```python
from build123d import *

# Parameters (mm, degrees)
SKETCH1_R               = 11
SKETCH1_R_2             = 5
SKETCH1_R_3             = 1.5
BOSS_EXTRUDE1_DEPTH     = 2
SKETCH1_3_R             = 5
SKETCH1_3_R_2           = 2
BOSS_EXTRUDE2_DEPTH     = 12
CUT_EXTRUDE1_REACH      = 25.759
CUT_EXTRUDE1_END_RADIUS = 2
SKETCH2_R               = 1.5


with BuildPart() as part:
    # Sketch1 → Boss-Extrude1 (new body)
    with BuildSketch(Plane(origin=(0, 0, 0), x_dir=(1, 0, 0), z_dir=(0, 1, 0))):
        with Locations(Location((0, 0, 0), (0, 0, 270))):
            Circle(SKETCH1_R)
        with Locations(Location((0, 0, 0), (0, 0, 270))):
            Circle(SKETCH1_R_2, mode=Mode.SUBTRACT)
        with Locations(Location((0, 8, 0), (0, 0, 270))):
            Circle(SKETCH1_R_3, mode=Mode.SUBTRACT)
        with Locations(Location((8, 0, 0), (0, 0, 270))):
            Circle(SKETCH1_R_3, mode=Mode.SUBTRACT)
        with Locations(Location((0, -8, 0), (0, 0, 270))):
            Circle(SKETCH1_R_3, mode=Mode.SUBTRACT)
        with Locations(Location((-8, 0, 0), (0, 0, 270))):
            Circle(SKETCH1_R_3, mode=Mode.SUBTRACT)
    extrude(amount=BOSS_EXTRUDE1_DEPTH)

    # Sketch1_3 → Boss-Extrude2 (add)
    with BuildSketch(Plane(origin=(0, 0, 0), x_dir=(1, 0, 0), z_dir=(0, 1, 0))):
        with Locations(Location((0, 0, 0), (0, 0, 270))):
            Circle(SKETCH1_3_R)
        with Locations(Location((0, 0, 0), (0, 0, 270))):
            Circle(SKETCH1_3_R_2, mode=Mode.SUBTRACT)
    extrude(amount=BOSS_EXTRUDE2_DEPTH)

    # Cut-Extrude1: up to this cylinder (the profile starts outside it)
    cut_extrude1_end = Plane(origin=(0, 9, 0), z_dir=(0, -1, 0)) * Cylinder(CUT_EXTRUDE1_END_RADIUS, 56.518, mode=Mode.PRIVATE)
    # Sketch2 → Cut-Extrude1 (cut, up to the surface)
    with BuildSketch(Plane(origin=(-4.0625, 0, 2.914805954), x_dir=(0.582961190817979, 0, 0.8125000000000517), z_dir=(-0.8125000000000517, 0, 0.582961190817979)), mode=Mode.PRIVATE) as cut_extrude1_sk1:
        with Locations((0, 9)):
            Circle(SKETCH2_R)
    cut_extrude1_tool1 = extrude(cut_extrude1_sk1.sketch, amount=-CUT_EXTRUDE1_REACH, mode=Mode.PRIVATE) - cut_extrude1_end
    add(cut_extrude1_tool1.solids().sort_by_distance((-4.0625, 9, 2.914806))[0], mode=Mode.SUBTRACT)


solid = part.part
```
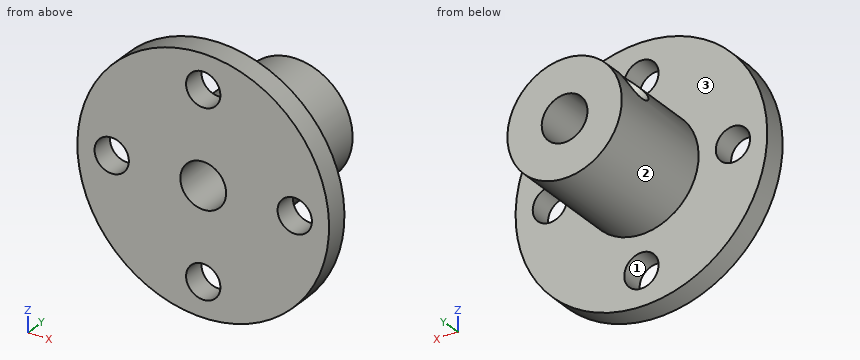
Can you work these out from the model? Positions are in its coordinate system, mm. Face numbers are marked on the shaded views. Coordinates: 2 decimals unless noted, no trailing zeros. Loops run counter-clockwise (first coordinate to the right, second up) from the corner with the lowest first, then second, coordinate; pieces in that order, holes last. Notation, with made-up numbers: M 59,-19 L 70,-19 A7 cw 70,-15 Z; hole C 46.25,50 d3. An arc over 180 degrees is marked long. Put each result on its own line as item: value. Start each with the question number.
(1) Imagine slicing it at A-A on x = 8. List the corners of the cut face in (y, z) for me, and give its area (3 significant figures).
(2) Imagine slicing it at B-B on z = 8. List the corners of the cut face in (x, y) for me, and give its area (3 significant figures).
(3) Imagine slicing it at C-C on y = 2.75. List the corners of the cut face in (x, z) for me, and give its area (3 significant figures).
(4) I need wall thicknesses on probe 1 along X at (y, z) = (1.05, 0); probe 2 along Y at (x, z) = (-5.5, 0.75); probe 3 along X at (y, z) = (0.4, 8). Which ranges of each line are inside material? Lowest first, please.
(5) Will these pins go through, and if not, where does the flat tip stop? pin 1 Ø3.5 at (x, z) = (0, 8) entering from +Y; pin 2 Ø4 at (x, y) = (-8, 2.5) entering from +Z; pin 3 Ø3 at (x, y) = (3, 10) entering from +Z.
(6) We'd pull the mould along X, two halves only. Please class the marked faces 1, 2 and 3: +X half, -X half, draft (parallel to the pull), parting line (faces both ways), or undercut.
(7) Imagine slicing it at D-D on z = -1. List the corners of the cut face in (x, y) for me.
Worked answers:
1. outline: M 0,-7.55 L 2,-7.55 L 2,-1.5 L 0,-1.5 Z; M 0,1.5 L 2,1.5 L 2,7.55 L 0,7.55 Z
1. area: 24.2 mm2
2. outline: M -7.55,0 L -1.5,0 L -1.5,2 L -7.55,2 Z; M 1.5,0 L 7.55,0 L 7.55,2 L 1.5,2 Z
2. area: 24.2 mm2
3. outline: C 0,0 d10; hole C 0,0 d4
3. area: 66.0 mm2
4. probe 1: x = -11 to -9.5, -6.5 to -2, 2 to 6.5, 9.5 to 11
4. probe 2: y = 0 to 2
4. probe 3: x = -7.55 to -1.5, 1.5 to 7.55
5. pin 1: stops at y = 2
5. pin 2: stops at z = 9.18
5. pin 3: stops at z = 4.77
6. face 1: undercut
6. face 2: parting line
6. face 3: draft
7. outline: M -10.95,0 L -9.12,0 L -9.12,2 L -10.95,2 Z; M -6.88,0 L -1.73,0 L -1.73,12 L -4.9,12 L -4.9,2 L -6.88,2 Z; M 1.73,0 L 6.88,0 L 6.88,2 L 4.9,2 L 4.9,12 L 1.73,12 Z; M 9.12,0 L 10.95,0 L 10.95,2 L 9.12,2 Z
